Verification items for this drawing (mm, ordinates from the low corner). A direction names the side the tool comes from. Round coordinates to 2 decimals unless told otherwise and drop trailing zeros. Write each loop counter-clockwise with the first axis right and the second up, starting at its lowest first coordinate (ties: lowest second). Pieces come first, ordered by that corner, then holes. Notation, with made-up numbers: (82.5, 18) -> (107.5, 18) arc R24 ccw to (107.5, 44) -> close; hole circle Ø2 at (53, 22.25). An arc over 180 degrees is marked (long way). One line per item, written item: value.
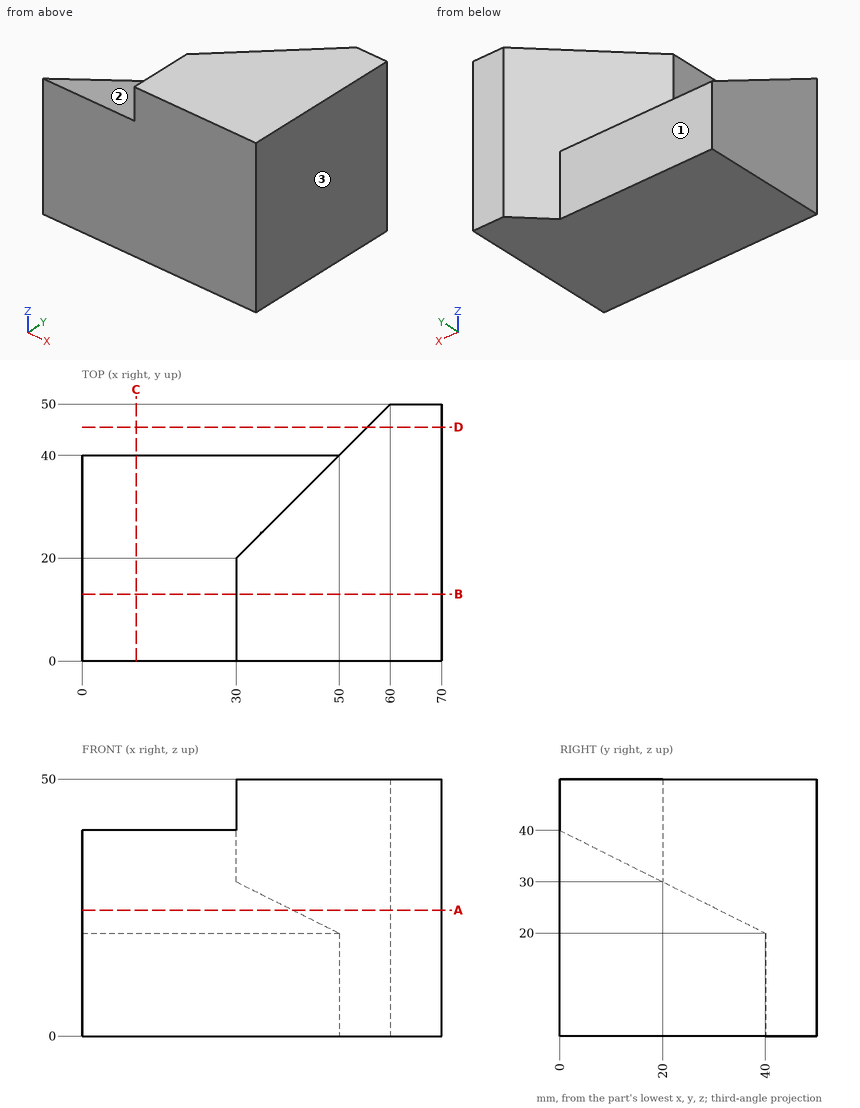
Item 1: Tool access check on the marked faces 1, 2 and 3. Record the directions out of +Z, -Z, +X, -X, +Y, -Y that give a thin tool (end or side, any length) a straight path to the whole face; none if there is none.
Result set:
face 1: +Z, -Z, -X, +Y
face 2: +Z, -X, +Y
face 3: +Z, -Z, +X, +Y, -Y
Item 2: Sectioned sample at C-C (x = 10.5). Enter the section's corners in (y, z).
Result set:
outline: (0, 0) -> (40, 0) -> (40, 20) -> (0, 40) -> close
Item 3: Material ranges on line 1 along Y through (x, z) = (8, 8); line 2 along X through (y, z) = (12.5, 47); line 3 along Y through (x, z) = (56, 13), recorded low to high.
Result set:
line 1: 0 to 40
line 2: 30 to 70
line 3: 0 to 46
Item 4: Sectioned sample at D-D (y = 45.5). Enter the section's corners in (x, z).
Result set:
outline: (55.5, 0) -> (70, 0) -> (70, 50) -> (55.5, 50) -> close
Item 5: Depth check by flat-ended pin: pin 1 (6 mm diameter, centred on x = 35, z = 14.5, fed in from +Y); pin 2 (10 mm diameter, centred on y = 13.5, z = 42, fed in from -X); pin 3 (12 mm diameter, centred on x = 41, z = 33.5, fed in from +Y). Enter the tip coordinate at first touch or a pass-through.
Result set:
pin 1: y = 40
pin 2: x = 30
pin 3: y = 37
Item 6: Sectioned sample at B-B (y = 13). Enter the section's corners in (x, z).
Result set:
outline: (0, 0) -> (70, 0) -> (70, 50) -> (30, 50) -> (30, 33.5) -> (0, 33.5) -> close
Item 7: Sectioned sample at A-A (z = 24.5). Enter the section's corners in (x, y), then the cut area to 3 significant figures.
Result set:
outline: (0, 0) -> (70, 0) -> (70, 50) -> (60, 50) -> (41, 31) -> (0, 31) -> close
area: 2,540 mm^2
